Source: CAD feature listing. Evaluate the final solid. Frame: model axes, mm. Face numbers are marked on the shaded views. A direction names the side the tool comes from. Round coordinates to 2 decimals unless told otherwise and drop trailing zeros. Loops run counter-clockwise (first coordinate to the right, second up) from the corner with the lowest first, then second, coordinate; pieces in that order, holes last. Notation, with made-up numbers: M 1,24 L 24,24 A23 ccw 24,50 Z; hole C -37.75,83.5 d3. An arc over 180 degrees is marked long. Answer as a JSON object with one key per item and string values.
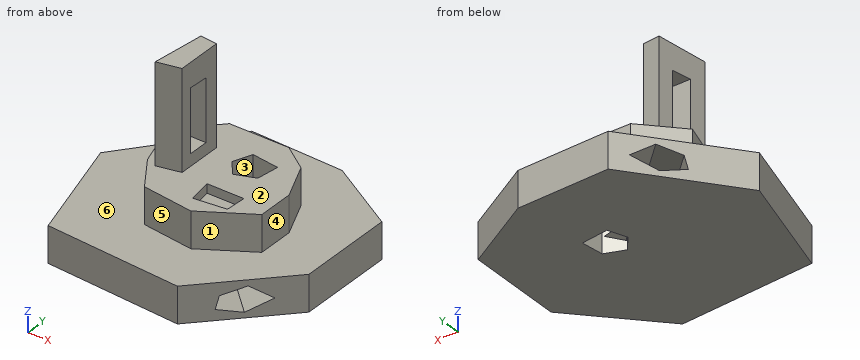
from build123d import *

# Parameters (mm, degrees)
PAD_DEPTH       = 20
PAD001_DEPTH    = 20
PAD002_DEPTH    = 55
POCKET_DEPTH    = 5
POCKET001_DEPTH = 40.001
POCKET002_DEPTH = 57.547898
POCKET003_DEPTH = 152.1407019841


with BuildPart() as part:
    # Sketch → Pad (new body)
    with BuildSketch(Plane.XY):
        Polygon((-20.459476, 40.117115), (31.15163, 38.233494), (70.707581, 14.876653), (70.707581, -39.371517), (29.644735, -82.317986), (-46.453392, -76.667137), (-63.782669, -14.507775), align=None)
    extrude(amount=PAD_DEPTH)

    # Sketch001 (on Face9 of Pad) → Pad001 (join)
    with BuildSketch(Plane.XY.offset(20)):
        Polygon((-13.537989, 14.137136), (19.591442, 14.137136), (33.855503, 4.014249), (43.058121, -17.151772), (43.058121, -37.397533), (15.910392, -53.96225), (-12.617725, -50.281197), (-25.041264, -31.415821), (-32.863491, -6.108627), align=None)
    extrude(amount=PAD001_DEPTH)

    # Sketch002 (on Face19 of Pad001) → Pad002 (join)
    with BuildSketch(Plane.XY.offset(40)):
        Polygon((-15.579205, -4.296096), (-6.235771, -5.306198), (-6.235771, -30.811253), (-19.114557, -33.589027), align=None)
    extrude(amount=PAD002_DEPTH)

    # Sketch003 (on Face19 of Pad002) → Pocket (cut)
    with BuildSketch(Plane.XY.offset(40)):
        Polygon((8.155688, -31.614529), (28.728765, -31.614529), (28.157293, -43.044018), (10.155849, -45.044178), align=None)
    extrude(amount=-POCKET_DEPTH, mode=Mode.SUBTRACT)

    # Sketch004 (on Face19 of Pocket) → Pocket001 (cut, through all)
    with BuildSketch(Plane.XY.offset(40)):
        Polygon((10.206862, 0), (25.338156, -1.995884), (23.614338, -14.445684), (12.696822, -18.467928), (6.184619, -10.42344), align=None)
    extrude(amount=-POCKET001_DEPTH, mode=Mode.SUBTRACT)

    # Sketch005 (on Face32 of Pocket001) → Pocket002 (cut, through all)
    with BuildSketch(Plane.YZ.offset(-6.235771)):
        Polygon((-24.452877, 81.538773), (-13.023387, 80.9673), (-13.023387, 46.678833), (-24.452877, 46.678833), align=None)
    extrude(amount=-POCKET002_DEPTH, mode=Mode.SUBTRACT)

    # Sketch006 (on Face9 of Pocket002) → Pocket003 (cut, through all)
    with BuildSketch(Plane(origin=(56.60434605, -54.1216914662, 0), x_dir=(0.6910786275, 0.7227795865, 0), z_dir=(0.7227795865, -0.6910786275, 0))):
        Polygon((-20.040229, 12.946631), (-7.015827, 16.777342), (5.050909, 9.115925), (-8.739645, 2.986793), (-21.955589, 5.859823), align=None)
    extrude(amount=-POCKET003_DEPTH, mode=Mode.SUBTRACT)


solid = part.part
Item 1: Section C-C on y = 7. Return the cut outline in (x, z).
Answer sheet:
{"outline": "M -46.72,0 L 70.71,0 L 70.71,20 L 29.65,20 L 29.65,40 L -20.35,40 L -20.35,20 L -46.72,20 Z; hole M -39.09,5.86 L -19.97,2.99 L -0.01,9.12 L -17.47,16.78 L -36.32,12.95 Z"}
Item 2: Section B-B on z = 27. Return the cut outline in (x, y), then the cut area to 3 significant figures.
Answer sheet:
{"outline": "M -32.86,-6.11 L -25.04,-31.42 L -12.62,-50.28 L 15.91,-53.96 L 43.06,-37.4 L 43.06,-17.15 L 33.86,4.01 L 19.59,14.14 L -13.54,14.14 Z; hole M 6.18,-10.42 L 12.7,-18.47 L 23.61,-14.45 L 25.34,-2 L 10.21,0 Z", "area": "3,740 mm²"}
Item 3: Line query: probe 1 along Z at (x, y) = (-7, -43); probe 2 along Z at (x, y) = (49, 7); probe 3 along Z at (x, y) = (-8.5, -19). Output: solid intervals per line, ascending. Write a range as from..to.
Answer sheet:
{"probe 1": "z = 0..40", "probe 2": "z = 0..20", "probe 3": "z = 0..5.35, 13.07..46.68, 81.27..95"}
Item 4: Contact query for flat-ended pins moving along their axis: pin 1 Ø11.5 at (x, z) = (-13.5, 60.5) entering from -Y; pin 2 Ø6 at (x, y) = (0, -55.5) entering from -Z; pin 3 Ø6 at (x, z) = (-13, 58) entering from +Y; pin 4 Ø6 at (y, z) = (16.5, 40) entering from +X. Output: stop coordinate, or through.
Answer sheet:
{"pin 1": "stops at y = -33.59", "pin 2": "stops at z = 0", "pin 3": "stops at y = -4.3", "pin 4": "stops at x = 20.49"}
Item 5: Pull-direction query (Y, two-part tool) for the marked faces 1, 2 and 3; classes: pulls with the +Y half, pulls with the -Y half, needs draft (parallel to the pull), parting line crosses it, or undercut.
Answer sheet:
{"face 1": "pulls with the -Y half", "face 2": "needs draft", "face 3": "undercut"}
Item 6: Access query for the marked faces 4, 5 and 6. Directions: +Z, -Z, +X, -X, +Y, -Y. A direction counts if a zero-diameter tool reaches every point of the face in a straight line with its end or side. Return the directions, or none.
Answer sheet:
{"face 4": "+Z, +X, +Y, -Y", "face 5": "+Z, -X, -Y", "face 6": "+Z"}
Item 7: Section D-D on x = 39.5. Return the cut outline in (y, z), then the cut area to 3 significant figures.
Answer sheet:
{"outline": "M -72.01,0 L 33.3,0 L 33.3,20 L -8.97,20 L -8.97,40 L -39.57,40 L -39.57,20 L -72.01,20 Z; hole M -68.14,5.86 L -49.86,2.99 L -30.78,9.12 L -47.47,16.78 L -65.49,12.95 Z", "area": "2,410 mm²"}
Item 8: Section A-A on z = 64. Return the cut outline in (x, y), then the cut area to 3 significant figures.
Answer sheet:
{"outline": "M -19.11,-33.59 L -6.24,-30.81 L -6.24,-24.45 L -18.01,-24.45 Z; M -16.63,-13.02 L -6.24,-13.02 L -6.24,-5.31 L -15.58,-4.3 Z", "area": "176 mm²"}
